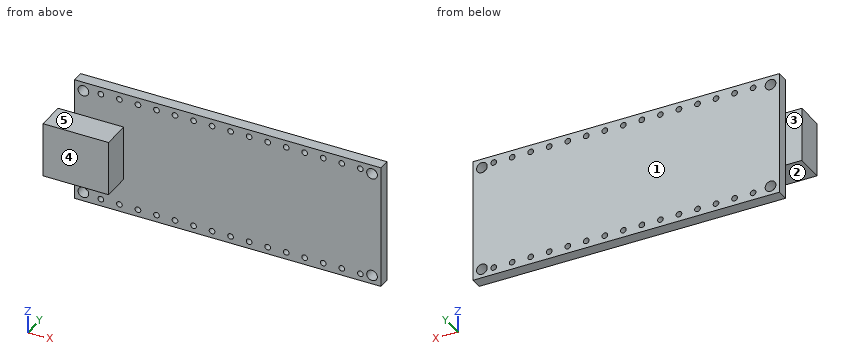
from build123d import *

# Parameters (mm, degrees)
F0_W     = 43
F0_H     = 17.5
F1_DEPTH = 1.6
F2_W     = 9.2
F2_H     = 7.7
F3_DEPTH = 4
F4_R     = 0.75
F5_DEPTH = 1.601
F6_R     = 0.4
F7_DEPTH = 1.601


with BuildPart() as f1:
    # F0 (on Front) → F1 (new body)
    with BuildSketch(Plane.XZ):
        Rectangle(F0_W, F0_H)
    extrude(amount=F1_DEPTH)

    # F2 (on face) → F3 (join)
    with BuildSketch(Plane.XZ.offset(1.6)):
        with Locations((-19.2, 0)):
            Rectangle(F2_W, F2_H)
    extrude(amount=F3_DEPTH)

    # F4 (on face) → F5 (cut, through all)
    with BuildSketch(Plane.XZ.offset(1.6)):
        with Locations((-20.25, 7.5)):
            Circle(F4_R)
        with Locations((-20.25, -7.5)):
            Circle(F4_R)
        with Locations((20.25, 7.5)):
            Circle(F4_R)
        with Locations((20.25, -7.5)):
            Circle(F4_R)
    extrude(amount=-F5_DEPTH, mode=Mode.SUBTRACT)

    # F6 (on face) → F7 (cut, through all)
    with BuildSketch(Plane.XZ.offset(1.6)):
        with Locations((-17.8, 7.75)):
            Circle(F6_R)
        with Locations((-15.2, 7.75)):
            Circle(F6_R)
        with Locations((-12.6, 7.75)):
            Circle(F6_R)
        with Locations((-10, 7.75)):
            Circle(F6_R)
        with Locations((-7.4, 7.75)):
            Circle(F6_R)
        with Locations((-4.8, 7.75)):
            Circle(F6_R)
        with Locations((-2.2, 7.75)):
            Circle(F6_R)
        with Locations((0.4, 7.75)):
            Circle(F6_R)
        with Locations((3, 7.75)):
            Circle(F6_R)
        with Locations((5.6, 7.75)):
            Circle(F6_R)
        with Locations((8.2, 7.75)):
            Circle(F6_R)
        with Locations((10.8, 7.75)):
            Circle(F6_R)
        with Locations((13.4, 7.75)):
            Circle(F6_R)
        with Locations((16, 7.75)):
            Circle(F6_R)
        with Locations((18.6, 7.75)):
            Circle(F6_R)
        with Locations((-17.8, -7.75)):
            Circle(F6_R)
        with Locations((-15.2, -7.75)):
            Circle(F6_R)
        with Locations((-12.6, -7.75)):
            Circle(F6_R)
        with Locations((0.4, -7.75)):
            Circle(F6_R)
        with Locations((-7.4, -7.75)):
            Circle(F6_R)
        with Locations((-4.8, -7.75)):
            Circle(F6_R)
        with Locations((-2.2, -7.75)):
            Circle(F6_R)
        with Locations((-10, -7.75)):
            Circle(F6_R)
        with Locations((18.6, -7.75)):
            Circle(F6_R)
        with Locations((16, -7.75)):
            Circle(F6_R)
        with Locations((13.4, -7.75)):
            Circle(F6_R)
        with Locations((5.6, -7.75)):
            Circle(F6_R)
        with Locations((3, -7.75)):
            Circle(F6_R)
        with Locations((8.2, -7.75)):
            Circle(F6_R)
        with Locations((10.8, -7.75)):
            Circle(F6_R)
    extrude(amount=-F7_DEPTH, mode=Mode.SUBTRACT)


solid = f1.part
Could you check a few things on this model? Use its own coordinates, in mm. Face numbers are marked on the shaded views. A direction names the side the tool comes from. Round coordinates to 2 decimals unless told otherwise and drop trailing zeros. Loops run counter-clockwise (first coordinate to the right, second up) from the corner with the lowest first, then second, coordinate; pieces in that order, holes last. Notation, with made-up numbers: (86.5, 36.5) -> (129.5, 36.5) arc R19 ccw to (129.5, 55.5) -> close; hole circle Ø5 at (31.5, -34.5). An arc over 180 degrees is marked (long way). Use CSV: the item, a comma, the result in double quotes.
(1) Suppose I cut it at A-A on x = 5.6. Write out the boundary of the cut face in (y, z).
Return value:
outline,"(-1.6, -8.75) -> (0, -8.75) -> (0, -8.15) -> (-1.6, -8.15) -> close; (-1.6, -7.35) -> (0, -7.35) -> (0, 7.35) -> (-1.6, 7.35) -> close; (-1.6, 8.15) -> (0, 8.15) -> (0, 8.75) -> (-1.6, 8.75) -> close"
(2) Suppose I cut it at C-C on y = -3.15. Write out the boundary of the cut face in (x, z).
Return value:
outline,"(-23.8, -3.85) -> (-14.6, -3.85) -> (-14.6, 3.85) -> (-23.8, 3.85) -> close"
(3) Suppose I cut it at D-D on y = -0.7. Give the number of separate pieces and of enclosed holes in the cut face, plus the area to 3 significant figures.
Return value:
separate pieces,"1"
enclosed holes,"34"
area,"730 mm²"
(4) If I drill on probe 1 along Z at (x, y) = (-20.25, -0.6); probe 2 along Z at (x, y) = (-10, -1); probe 3 along Y at (x, z) = (-19, -8), over which ranges is the centre line in solid material (lowest first)? Write a range as [from, to].
Return value:
probe 1,"z = [-8.75, -8.25], [-6.75, 6.75], [8.25, 8.75]"
probe 2,"z = [-8.75, -8.15], [-7.35, 7.35], [8.15, 8.75]"
probe 3,"y = [-1.6, 0]"
(5) Suppose I cut it at B-B on z = 3.25. Write out the boundary of the cut face in (x, y).
Return value:
outline,"(-23.8, -5.6) -> (-14.6, -5.6) -> (-14.6, -1.6) -> (21.5, -1.6) -> (21.5, 0) -> (-21.5, 0) -> (-21.5, -1.6) -> (-23.8, -1.6) -> close"
(6) Will these pins go through, and if not, where does the flat tip stop? pin 1 Ø9 at (x, z) = (-2, -1) entering from -Y; pin 2 Ø1.2 at (x, y) = (-18, -3) entering from +Z; pin 3 Ø4 at (x, z) = (-14, -3.5) entering from -Y; pin 4 Ø1.8 at (y, z) = (-0.5, 2) entering from -X.
Return value:
pin 1,"stops at y = -1.6"
pin 2,"stops at z = 3.85"
pin 3,"stops at y = -5.6"
pin 4,"stops at x = -21.5"
(7) For the marked faces 1, 2, 3, 4 and 5, which set-ups out of +Z, -Z, +X, -X, +Y, -Y let a thin tool reach every point of the face, with its end or its side?
Return value:
face 1,"+Z, -Z, +X, -X, +Y"
face 2,"-Z, +X, -X, -Y"
face 3,"+Z, -Z, -X, +Y"
face 4,"+Z, -Z, +X, -X, -Y"
face 5,"+Z, +X, -X, -Y"
